from build123d import *

# Parameters (mm, degrees)
SKETCH1_R                                           = 60.625
SKETCH1_R_2                                         = 45
BOSS_EXTRUDE1_DEPTH                                 = 4
SKETCH2_R                                           = 49
SKETCH2_R_2                                         = 45
BOSS_EXTRUDE2_DEPTH                                 = 52
SKETCH4_W                                           = 13.25
SKETCH4_H                                           = 8
SKETCH4_W_2                                         = 8
SKETCH4_H_2                                         = 38
BOSS_EXTRUDE4_DEPTH                                 = 13
BOSS_EXTRUDE5_DEPTH                                 = 4
SKETCH7_R                                           = 1.3
CUT_EXTRUDE4_DEPTH                                  = 39
SKETCH9_W                                           = 10
SKETCH9_H                                           = 24
CUT_EXTRUDE7_DEPTH                                  = 8
CUT_EXTRUDE9_DEPTH                                  = 5
CSK_FOR_M3_COUNTERSUNK_FLAT_HEAD_SCREW1_D           = 3.4
CSK_FOR_M3_COUNTERSUNK_FLAT_HEAD_SCREW1_DEPTH       = 4
CSK_FOR_M3_COUNTERSUNK_FLAT_HEAD_SCREW1_CSINK_D     = 6.3
CSK_FOR_M3_COUNTERSUNK_FLAT_HEAD_SCREW1_CSINK_ANGLE = 90


with BuildPart() as part:
    # Sketch1 → Boss-Extrude1 (new body)
    with BuildSketch(Plane(origin=(0, 0, 0), x_dir=(1, 0, 0), z_dir=(0, 1, 0))):
        Circle(SKETCH1_R)
        Circle(SKETCH1_R_2, mode=Mode.SUBTRACT)
    extrude(amount=BOSS_EXTRUDE1_DEPTH)

    # Sketch2 → Boss-Extrude2 (add)
    with BuildSketch(Plane(origin=(0, 4, 0), x_dir=(1, 0, 0), z_dir=(0, 1, 0))):
        Circle(SKETCH2_R)
        Circle(SKETCH2_R_2, mode=Mode.SUBTRACT)
    extrude(amount=BOSS_EXTRUDE2_DEPTH)

    # Sketch4 → Boss-Extrude4 (add, symmetric)
    with BuildSketch(Plane.XY):
        with Locations((-38.375, 34)):
            Rectangle(SKETCH4_W, SKETCH4_H)
        Polygon((-31.75, 30), (-45, 30), (-45, 16.75), align=None)
        with Locations((15.25, 19)):
            Rectangle(SKETCH4_W_2, SKETCH4_H_2)
    extrude(amount=BOSS_EXTRUDE4_DEPTH, both=True)

    # Sketch5 → Boss-Extrude5 (add)
    with BuildSketch(Plane.XZ):
        with BuildLine():
            Line((11.25, 13), (29.067400866, 34.352382842))
            ThreePointArc((29.067400866, 34.352382842), (45, 0), (29.067400866, -34.352382842))
            Line((29.067400866, -34.352382842), (11.25, -13))
            Line((11.25, -13), (11.25, 13))
        make_face()
    extrude(amount=-BOSS_EXTRUDE5_DEPTH)

    # Sketch7 → Cut-Extrude4 (cut, through all)
    with BuildSketch(Plane(origin=(0, 38, 0), x_dir=(1, 0, 0), z_dir=(0, 1, 0))):
        with Locations((-34.25, 5)):
            Circle(SKETCH7_R)
        with Locations((-34.25, -5)):
            Circle(SKETCH7_R)
        with Locations((13.75, 5)):
            Circle(SKETCH7_R)
        with Locations((13.75, -5)):
            Circle(SKETCH7_R)
    extrude(amount=-CUT_EXTRUDE4_DEPTH, mode=Mode.SUBTRACT)

    # Sketch9 → Cut-Extrude7 (cut)
    with BuildSketch(Plane.ZY.offset(-11.25)):
        with Locations((0, 17)):
            Rectangle(SKETCH9_W, SKETCH9_H)
    extrude(amount=-CUT_EXTRUDE7_DEPTH, mode=Mode.SUBTRACT)

    # Sketch12 → Cut-Extrude9 (cut, through all)
    with BuildSketch(Plane(origin=(0, 4, 0), x_dir=(1, 0, 0), z_dir=(0, 1, 0))):
        with BuildLine():
            Line((29.479537487, 22.359715328), (27.25, 19.687836398))
            Line((27.25, 19.687836398), (27.25, -19.687836398))
            Line((27.25, -19.687836398), (29.479537487, -22.359715328))
            ThreePointArc((29.479537487, -22.359715328), (37, 0), (29.479537487, 22.359715328))
        make_face()
        Polygon((27.25, -19.687836398), (27.25, 19.687836398), (24.25, 16.092634774), (24.25, -16.092634774), align=None)
    extrude(amount=-CUT_EXTRUDE9_DEPTH, mode=Mode.SUBTRACT)

    # CSK for M3 Countersunk Flat Head Screw1
    with Locations(Plane(origin=(0, 4, 0), x_dir=(1, 0, 0), z_dir=(0, 1, 0))):
        with Locations((-38.890872965, 38.890872965), (-38.890872965, -38.890872965), (38.890872965, -38.890872965), (38.890872965, 38.890872965)):
            CounterSinkHole(CSK_FOR_M3_COUNTERSUNK_FLAT_HEAD_SCREW1_D / 2, CSK_FOR_M3_COUNTERSUNK_FLAT_HEAD_SCREW1_CSINK_D / 2, depth=CSK_FOR_M3_COUNTERSUNK_FLAT_HEAD_SCREW1_DEPTH, counter_sink_angle=CSK_FOR_M3_COUNTERSUNK_FLAT_HEAD_SCREW1_CSINK_ANGLE)


solid = part.part
Can you work these out from the model? Positions are in its coordinate system, mm. A direction names the side the tool comes from. Round coordinates to 2 decimals unless told otherwise and drop trailing zeros. Loops run counter-clockwise (first coordinate to the right, second up) from the corner with the lowest first, then second, coordinate; pieces in that order, holes last. Notation, with made-up numbers: (-39.75, -15.75) - (0.25, -15.75) arc R19 ccw to (0.25, 21.25) - close; hole circle Ø1 at (-38, 32.5). An arc over 180 degrees is marked (long way). Write item = value, one per line. Start each with the question number.
(1) If I drill on probe 1 along X at (y, z) = (42, 0); probe 2 along X at (y, z) = (34.5, 0); probe 3 along Z at (x, y) = (-34, 35), over which ranges is the centre line in solid material (lowest first)? Write a range as [from, to].
(2) If we section it at C-C (z = 0): Please give me the cut outline in (x, y) (3 decimals), and give its area (3 significant figures).
(3) For faces 4 (the face through (17, 17, -5)), 5 (the face through (-39, 31, -13)), 6 (the face through (19.25, 21, 6)), which set-ups out of +Z, -Z, +X, -X, +Y, -Y let a thin tool reach every point of the face, with its end or its side?
(4) If we section it at B-B (y = 23.5): Please give me the cut outline in (x, z).
(5) If we section it at A-A (y = 31.5): Please give me the cut outline in (x, z).
(6) For P1, Ø9, axis at x = -37, y = 26, coming from the -Z side; P2, Ø4, axis at x = -34.25, z = -5, coming from the -Y side; P3, Ø4, axis at x = 13.75, z = -5, coming from the -Y side; P4, Ø4, axis at x = 38.89, z = -38.89, coming from the +Y side, each with a flat end and sliding along its axis, tell me the tip position at first contact or that it passes through.
(7) If we section it at D-D (x = 0): Please give me the cut outline in (y, z) (3 decimals).
(8) If we mould it in two halves opening along Y, with no side actions, what happens to faces 1 (the face through (20.283, 1.972, -23.826)), 2 (the face through (15, 29, 0)), 3 (the face through (-5, 4, 49))? For each: released by +Y, released by -Y, zero draft, split by the parting line, or undercut.
Ans:
q1.probe_1 = [-49, -45], [45, 49]
q1.probe_2 = [-49, -31.75], [11.25, 19.25], [45, 49]
q1.probe_3 = [-35.28, -29.48], [-13, -6.28], [-3.72, 3.72], [6.28, 13], [29.48, 35.28]
q2.outline = (-60.625, 0) - (-45, 0) - (-45, 16.75) - (-31.75, 30) - (-31.75, 38) - (-45, 38) - (-45, 56) - (-49, 56) - (-49, 4) - (-60.625, 4) - close; (11.25, 0) - (24.25, 0) - (24.25, 4) - (19.25, 4) - (19.25, 5) - (11.25, 5) - close; (11.25, 29) - (19.25, 29) - (19.25, 38) - (11.25, 38) - close; (37, 0) - (60.625, 0) - (60.625, 4) - (49, 4) - (49, 56) - (45, 56) - (45, 4) - (37, 4) - close
q2.area = 899 mm²
q3.face_4 = none
q3.face_5 = +Y, -Y
q3.face_6 = +Y
q4.outline = circle Ø98 at (0, 0); (11.25, -13) - (19.25, -13) - (19.25, -5) - (15.05, -5) arc R1.3 cw to (12.45, -5) - (11.25, -5) - close; (11.25, 5) - (12.45, 5) arc R1.3 cw to (15.05, 5) - (19.25, 5) - (19.25, 13) - (11.25, 13) - close; hole (-43.08, -13) arc R45 ccw (long way) to (-43.08, 13) - (-38.25, 13) - (-38.25, -13) - close
q5.outline = circle Ø98 at (0, 0); (11.25, -13) - (19.25, -13) - (19.25, 13) - (11.25, 13) - close; hole (-43.08, -13) arc R45 ccw (long way) to (-43.08, 13) - (-31.75, 13) - (-31.75, -13) - close; hole circle Ø2.6 at (-34.25, -5); hole circle Ø2.6 at (-34.25, 5); hole circle Ø2.6 at (13.75, -5); hole circle Ø2.6 at (13.75, 5)
q6.P1 = -36.67
q6.P2 = 25.5
q6.P3 = 0
q6.P4 = 2.85
q7.outline = (0, -60.625) - (4, -60.625) - (4, -49) - (56, -49) - (56, -45) - (0, -45) - close; (0, 45) - (56, 45) - (56, 49) - (4, 49) - (4, 60.625) - (0, 60.625) - close
q8.face_1 = zero draft
q8.face_2 = undercut
q8.face_3 = released by +Y
